Geometry check sheet. Reference: drawing and pictorial views, mm from the part's lowest x, y, z. A direction names the side the tool comes from. Round coordinates to 2 decimals unless told otherwise and drop trailing zeros. Order: outer loops, then holes, each group sorted by start corner. A loop starts at its lowest first (then second) coordinate and runs counter-clockwise, first axis right, second up.
(1) Set-up check for the marked faces 1, 2 and 3: record each of +Z, -Z, +X, -X, +Y, -Y from which the full face is reachable in a straight line by a thin tool's end or side.
(2) Sectioned sample at A-A (x = 6). Record the boundary of the cut face in (y, z).
(3) Go/stop test with flat-tipped pins: pin 1 (1.5 mm diameter, centred on x = 18.5, z = 3, fed in from -Y); pin 2 (10 mm diameter, centred on x = 6.5, y = 21.5, fed in from +Z); pin 3 (0.7 mm diameter, centred on x = 32, z = 2, fed in from -Y). Record where each tip stops, or that it passes through.
(4) Release check for a two-part mould opening along X. For the marked faces 4, 5, 6 and 7 record: +X half, -X half, draft (parallel to the pull), parting line (faces both ways), or undercut.
(5) Material ranges on line 1 along Z through (x, y) = (23.5, 1.75); line 2 along X through (y, z) = (15.5, 2.25) (1 decimal); line 3 along Y through (x, z) = (19.5, 4.5) (1 decimal), recorded low to high.
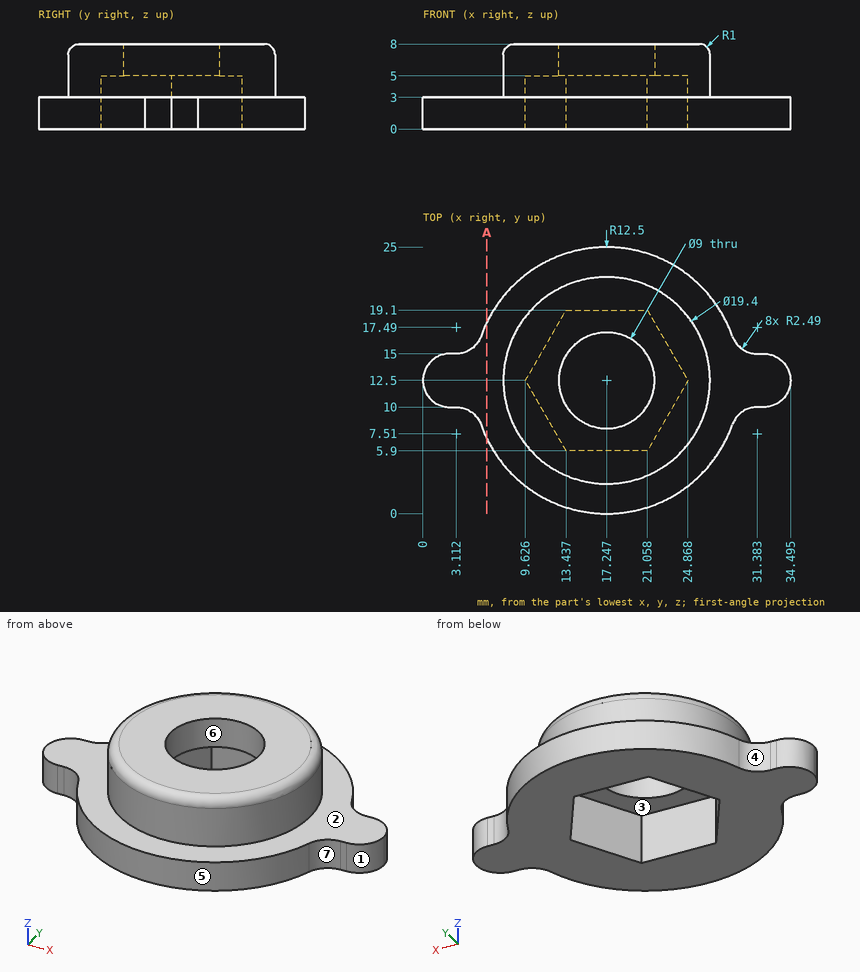
Answer below:
1. face 1: +Z, -Z, +X, -Y
1. face 2: +Z
1. face 3: -Z
2. outline: (7.05, 0) - (17.95, 0) - (17.95, 3) - (7.05, 3) - close
3. pin 1: stops at y = 0.01
3. pin 2: stops at z = 7.95
3. pin 3: stops at y = 10
4. face 4: -X half
4. face 5: parting line
4. face 6: undercut
4. face 7: +X half
5. line 1: z = 0 to 3
5. line 2: x = 4.6 to 11.4, 23.1 to 29.9
5. line 3: y = 3.1 to 5.9, 19.1 to 21.9
